```python
from build123d import *

# Parameters (mm, degrees)
F0_W     = 2.5
F0_H     = 6
F1_DEPTH = 90
F2_R     = 2.25
F3_DEPTH = 25
F4_R     = 2.99999
F5_R     = 2.25
F6_DEPTH = 25
F7_R     = 2.99999


# Not quite as in the source:
# - a fillet or chamfer is up to 0.001 mm smaller than in the source, because OpenCascade refuses the exact size


with BuildPart() as f1:
    # F0 (on Front) → F1 (new body)
    with BuildSketch(Plane.XZ):
        Rectangle(F0_W, F0_H)
    extrude(amount=F1_DEPTH)

    # F2 (on face) → F3 (cut)
    with BuildSketch(Plane(origin=(-1.25, 0, 0), x_dir=(0, -1, 0), z_dir=(-1, 0, 0))):
        with Locations((3, 0)):
            Circle(F2_R)
    extrude(amount=-F3_DEPTH, mode=Mode.SUBTRACT)

    # F4 (radius 3 in the source; OpenCascade refuses exactly that, so slightly less here)
    f4_edges = [f1.edges().sort_by_distance(p)[0] for p in [
        (0, 0, 3),
        (0, 0, -3),
    ]]
    fillet(f4_edges, radius=F4_R)

    # F5 (on face) → F6 (cut)
    with BuildSketch(Plane(origin=(-1.25, 0, 0), x_dir=(0, -1, 0), z_dir=(-1, 0, 0))):
        with Locations((87, 0.2363782405)):
            Circle(F5_R)
    extrude(amount=-F6_DEPTH, mode=Mode.SUBTRACT)

    # F7 (radius 3 in the source; OpenCascade refuses exactly that, so slightly less here)
    f7_edges = [f1.edges().sort_by_distance(p)[0] for p in [
        (0, -90, 3),
        (0, -90, -3),
    ]]
    fillet(f7_edges, radius=F7_R)


solid = f1.part
```
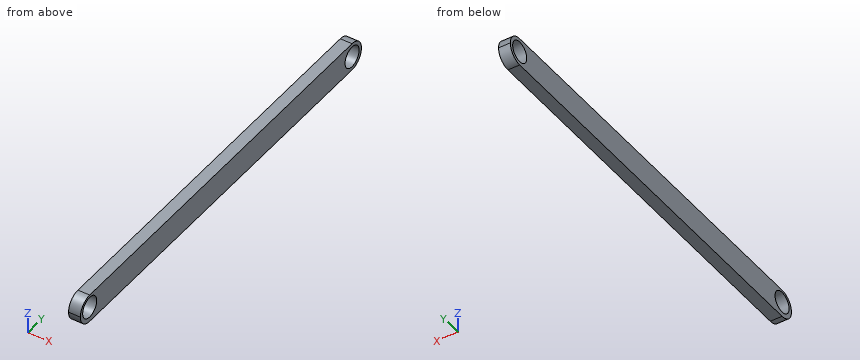
The model under review builds one solid part; all positions refer to its coordinate system, in mm. Give positions to 0.01 mm unless a question says otherwise; leave off trailing zeros. Write each loop counter-clockwise with the first axis right and the second up, starting at its lowest first coordinate (ties: lowest second). Pieces come first, ordered by that corner, then holes.
(1) To check wall thickness, follow L1, parallel to Z at x = -0.1, y = -87; L2, parallel to Y at x = 0.6, z = -0.25; L3, parallel to Y at x = -0.4, z = 1. State the ranges of each line that lie inside material, in increasing order.
(2) For P1, Ø2.5, axis at y = -87, z = 0.24, coming from the +X side, flat-tipped, find the tip position at first contact; note if it passes through.
(3) Consider section B-B, the plane x = -0.8. Give the number of separate pieces and of enclosed holes in the cut face, and give its area (3 significant figures).
(4) Consider section A-A, the plane z = 1. Give the boundary of the cut face in (x, y), and give its area (3 significant figures).
Returned:
1. L1: z = -3 to -2.01, 2.49 to 3
1. L2: y = -89.99 to -89.2, -84.8 to -5.24, -0.76 to -0.01
1. L3: y = -89.83 to -89.12, -84.88 to -5.02, -0.98 to -0.17
2. P1: passes through
3. separate pieces: 1
3. enclosed holes: 2
3. area: 500 mm2
4. outline: (-1.25, -89.83) - (1.25, -89.83) - (1.25, -89.12) - (-1.25, -89.12) - close; (-1.25, -84.88) - (1.25, -84.88) - (1.25, -5.02) - (-1.25, -5.02) - close; (-1.25, -0.98) - (1.25, -0.98) - (1.25, -0.17) - (-1.25, -0.17) - close
4. area: 203 mm2
